The listing builds one solid part. Answer for the finished solid, in the listing's coordinates (mm). Give positions to 0.01 mm unless a question says otherwise; leave off trailing zeros. Loops run counter-clockwise (first coordinate to the right, second up) from the corner with the lowest first, then second, coordinate; pieces in that order, holes last. Notation, with made-up numbers: (-29, 13.25) - (24, 13.25) arc R11 cw to (24, 20.25) - close; hole circle Ø9 at (42, 77). An arc over 180 degrees is marked (long way). Answer as CSV lines item,"result". Start each with the question number.
1) A cutting plane is placed at C-C (y = -1.15). Give the number of separate pieces and of enclosed holes in the cut face, and give its area (3 significant figures).
2) A cutting plane is placed at A-A (x = 107.95). Determine the outline of the cut face in (y, z).
3) For a pull along X with two mould halves and no side action, classify faces 1 (the face through (106, -1.524, -56)), 2 (the face through (3.82, -0.75, -3.62)), 3 (the face through (10.628, -0.751, -11.633)) as pulls with the +X half, pulls with the -X half, needs draft (parallel to the pull), parting line crosses it, or undercut.
4) Find the intervals of material crossed by line 1 along X through (y, z) = (-0.75, -57.15); line 2 along Z through (x, y) = (107.95, -0.6); line 3 along X through (y, z) = (-0.35, -10), in increasing order.
5) A flat-ended cylindrical pin translates along its axis: pin 1 (2.5 mm diameter, centred on x = 107.95, z = -104.775, fed in from -Y). Find the tip coordinate at first contact, or state that the pin passes through.
6) A cutting plane is placed at B-B (x = 144). Determine the outline of the cut face in (y, z) (3 decimals).
7) A cutting plane is placed at D-D (x = 205.74). Determine the outline of the cut face in (y, z), and give its area (3 significant figures).
```python
from build123d import *

# Parameters (mm, degrees)
F1_DEPTH = 1.524
F3_DEPTH = 1.525
F5_D     = 4.318


with BuildPart() as f1:
    # F0 (on Front) → F1 (new body)
    with BuildSketch(Plane.XZ):
        with BuildLine():
            Line((203.2, 0), (12.7, 0))
            ThreePointArc((12.7, 0), (3.7197438789, -3.7197438789), (0, -12.7))
            Line((0, -12.7), (0, -101.6))
            ThreePointArc((0, -101.6), (3.7197438789, -110.5802561211), (12.7, -114.3))
            Line((12.7, -114.3), (203.2, -114.3))
            ThreePointArc((203.2, -114.3), (212.1802561211, -110.5802561211), (215.9, -101.6))
            Line((215.9, -101.6), (215.9, -12.7))
            ThreePointArc((215.9, -12.7), (212.1802561211, -3.7197438789), (203.2, 0))
        make_face()
    extrude(amount=F1_DEPTH)

    # F2 (on face) → F3 (cut, through all)
    with BuildSketch(Plane.XZ.offset(1.524)):
        with BuildLine():
            ThreePointArc((61.9608133082, -66.0217711207), (63.5, -65.3542), (65.0391866918, -66.0217711207))
            ThreePointArc((65.0391866918, -66.0217711207), (63.5, -48.1457), (61.9608133082, -66.0217711207))
        make_face()
        with BuildLine():
            ThreePointArc((157.1370459911, -62.865), (159.2595306783, -62.0924787512), (160.3888811915, -60.1363862827))
            Line((160.3888811915, -60.1363862827), (160.6467393494, -58.674))
            Line((160.6467393494, -58.674), (163.576, -58.674))
            ThreePointArc((163.576, -58.674), (165.1, -57.15), (163.576, -55.626))
            Line((163.576, -55.626), (161.1841839866, -55.626))
            Line((161.1841839866, -55.626), (161.2398352004, -55.3103862827))
            ThreePointArc((161.2398352004, -55.3103862827), (160.5174787512, -52.6145153128), (157.988, -51.435))
            Line((157.988, -51.435), (135.8392, -51.435))
            ThreePointArc((135.8392, -51.435), (133.3097212488, -52.6145153128), (132.5873647996, -55.3103862827))
            Line((132.5873647996, -55.3103862827), (132.6430160134, -55.626))
            Line((132.6430160134, -55.626), (130.2512, -55.626))
            ThreePointArc((130.2512, -55.626), (128.7272, -57.15), (130.2512, -58.674))
            Line((130.2512, -58.674), (133.1804606506, -58.674))
            Line((133.1804606506, -58.674), (133.4383188085, -60.1363862827))
            ThreePointArc((133.4383188085, -60.1363862827), (134.5676693217, -62.0924787512), (136.6901540089, -62.865))
            Line((136.6901540089, -62.865), (157.1370459911, -62.865))
        make_face()
    extrude(amount=-F3_DEPTH, mode=Mode.SUBTRACT)

    # F5 (through all)
    with Locations(Plane.XZ.offset(1.524)):
        with Locations((10.16, -9.525), (107.95, -9.525), (205.74, -9.525), (205.74, -104.775), (107.95, -104.775), (10.16, -104.775)):
            Hole(F5_D / 2)


solid = f1.part
```
Ans:
1,separate pieces,"1"
1,enclosed holes,"8"
1,area,"23,900 mm2"
2,outline,"(-1.52, -114.3) - (0, -114.3) - (0, -106.93) - (-1.52, -106.93) - close; (-1.52, -102.62) - (0, -102.62) - (0, -11.68) - (-1.52, -11.68) - close; (-1.52, -7.37) - (0, -7.37) - (0, 0) - (-1.52, 0) - close"
3,face 1,"needs draft"
3,face 2,"pulls with the -X half"
3,face 3,"undercut"
4,line 1,"0 to 54.5, 72.5 to 128.73, 165.1 to 215.9"
4,line 2,"-114.3 to -106.93, -102.62 to -11.68, -7.37 to 0"
4,line 3,"0.29 to 8.05, 12.27 to 105.84, 110.06 to 203.63, 207.85 to 215.61"
5,pin 1,"through"
6,outline,"(-1.524, -114.3) - (0, -114.3) - (0, -62.865) - (-1.524, -62.865) - close; (-1.524, -51.435) - (0, -51.435) - (0, 0) - (-1.524, 0) - close"
7,outline,"(-1.52, -114.04) - (0, -114.04) - (0, -106.93) - (-1.52, -106.93) - close; (-1.52, -102.62) - (0, -102.62) - (0, -11.68) - (-1.52, -11.68) - close; (-1.52, -7.37) - (0, -7.37) - (0, -0.26) - (-1.52, -0.26) - close"
7,area,"160 mm2"
